```python
from build123d import *

# Parameters (mm, degrees)
SKETCH1_W           = 82
SKETCH1_H           = 82
BOSS_EXTRUDE3_DEPTH = 4
SKETCH6_W           = 10
SKETCH6_H           = 4
BOSS_EXTRUDE4_DEPTH = 12
CIRPATTERN1_COUNT   = 3
CIRPATTERN1_ANGLE   = 180
SKETCH8_W           = 4
SKETCH8_H           = 10
BOSS_EXTRUDE5_DEPTH = 85
SKETCH12_W          = 15.333160426
SKETCH12_H          = 4
BOSS_EXTRUDE6_DEPTH = 33
SKETCH9_W           = 7
SKETCH9_H           = 7
BOSS_EXTRUDE7_DEPTH = 4
SKETCH13_W          = 7
SKETCH13_H          = 7
BOSS_EXTRUDE8_DEPTH = 4


with BuildPart() as part:
    # Sketch1 → Boss-Extrude3 (new body)
    with BuildSketch(Plane.XY):
        Rectangle(SKETCH1_W, SKETCH1_H)
    extrude(amount=BOSS_EXTRUDE3_DEPTH)

    # Sketch6 → Boss-Extrude4 (add)
    with BuildSketch(Plane(origin=(0, 41, 0), x_dir=(1, 0, 0), z_dir=(0, 1, 0))):
        with Locations((0, -2)):
            Rectangle(SKETCH6_W, SKETCH6_H)
    boss_extrude4 = extrude(amount=BOSS_EXTRUDE4_DEPTH)

    # CirPattern1: Boss-Extrude4 ×3 about axis
    cirpattern1_axis = Axis((0, 0, 0), (0, 0, -1))
    for i in range(1, CIRPATTERN1_COUNT):
        add(boss_extrude4.rotate(cirpattern1_axis, i * CIRPATTERN1_ANGLE / (CIRPATTERN1_COUNT - 1)))

    # Sketch8 → Boss-Extrude5 (add)
    with BuildSketch(Plane.ZY.offset(41)):
        with Locations((2, 0)):
            Rectangle(SKETCH8_W, SKETCH8_H)
    extrude(amount=BOSS_EXTRUDE5_DEPTH)

    # Sketch12 → Boss-Extrude6 (add)
    with BuildSketch(Plane(origin=(0, 5, 0), x_dir=(1, 0, 0), z_dir=(0, 1, 0))):
        with Locations((-96, -2)):
            Rectangle(SKETCH12_W, SKETCH12_H)
    boss_extrude6 = extrude(amount=BOSS_EXTRUDE6_DEPTH)

    # Sketch9 → Boss-Extrude7 (add)
    with BuildSketch(Plane.XY.offset(4)):
        with Locations((-96, 0)):
            Rectangle(SKETCH9_W, SKETCH9_H)
    extrude(amount=BOSS_EXTRUDE7_DEPTH)

    # Sketch13 → Boss-Extrude8 (add)
    with BuildSketch(Plane.XY.offset(4)):
        with Locations((-96, 23.5)):
            Rectangle(SKETCH13_W, SKETCH13_H)
    boss_extrude8 = extrude(amount=BOSS_EXTRUDE8_DEPTH)

    # Mirror2: Boss-Extrude6, Boss-Extrude8 across plane
    add(boss_extrude6.mirror(Plane(origin=(0, 0, 0), x_dir=(0, 0, 1), z_dir=(0, -1, 0))))
    add(boss_extrude8.mirror(Plane(origin=(0, 0, 0), x_dir=(0, 0, 1), z_dir=(0, -1, 0))))


solid = part.part
```
Model file for the job. Use its own axes, mm. A direction names the side the tool comes from. Coordinates: 2 decimals unless noted, no trailing zeros. Order: outer loops, then holes, each group sorted by start corner. A loop starts at its lowest first (then second) coordinate and runs counter-clockwise, first axis right, second up. Notation, with made-up numbers: (25.5, -25.75) - (84.5, -25.75) arc R8 ccw to (84.5, -11.75) - close; hole circle Ø10 at (-23, 35). An arc over 180 degrees is marked (long way). Return JSON: item names as keys, results as strings. Group by question number.
1) Probe line 1 (Y direction, x = -94, z = 4.5); line 2 (X direction, y = -15, z = 3); line 3 (Z direction, x = -32.5, y = 26.5). List the from-to ranges inside material, lowest first. Write a range as from..to.
2) Flat gauge pins, fed straight in: P1, Ø3, axis at x = 9, z = 3.5, coming from the -Y side; P2, Ø4.5, axis at y = -15.5, z = 2, coming from the +X side; P3, Ø2, axis at y = -28.5, z = 1.5, coming from the -X side; P4, Ø3, axis at y = 38.5, z = 6, coming from the -X side. Where does each tip first touch, or does it go through?
3) Saw through at B-B, the plane z = 5.5. Write the cut outline in (x, y).
4) Saw through at D-D, the plane x = -94.5. Write the cut outline in (y, z), plus the area to 3 significant figures.
5) Mould opens along Y. For faces 1 (the flat face through (23, 41, 2)), 2 (the flat face through (-96, -20, 6)), 3 (the flat face through (-126, 0, 2)) say: released by +Y, released by -Y, zero draft, split by the parting line, or undercut.
6) Saw through at C-C, the plane y = -1.5. Write the cut outline in (x, z), plus the area to 3 significant figures.
7) Tool access for faces 4 (the flat face through (-99.5, -23, 6)), 5 (the flat face through (-96, 3.5, 6)), 6 (the flat face through (-5, 47, 2)): list every direction of +Z, -Z, +X, -X, +Y, -Y with a clear straight run to the whole face (end or side of a thin tool).
8) Saw through at A-A, the plane y = 11.5. Write the cut outline in (x, z).
Values found:
{
 "1": {"line 1": "y = -27..-20, -3.5..3.5, 20..27", "line 2": "x = -103.67..-88.33, -41..41", "line 3": "z = 0..4"},
 "2": {"P1": "stops at y = -41", "P2": "stops at x = 41", "P3": "stops at x = -103.67", "P4": "passes through"},
 "3": {"outline": "(-99.5, -27) - (-92.5, -27) - (-92.5, -20) - (-99.5, -20) - close; (-99.5, -3.5) - (-92.5, -3.5) - (-92.5, 3.5) - (-99.5, 3.5) - close; (-99.5, 20) - (-92.5, 20) - (-92.5, 27) - (-99.5, 27) - close"},
 "4": {"outline": "(-38, 0) - (38, 0) - (38, 4) - (27, 4) - (27, 8) - (20, 8) - (20, 4) - (3.5, 4) - (3.5, 8) - (-3.5, 8) - (-3.5, 4) - (-20, 4) - (-20, 8) - (-27, 8) - (-27, 4) - (-38, 4) - close", "area": "388 mm²"},
 "5": {"face 1": "released by +Y", "face 2": "undercut", "face 3": "zero draft"},
 "6": {"outline": "(-126, 0) - (53, 0) - (53, 4) - (-92.5, 4) - (-92.5, 8) - (-99.5, 8) - (-99.5, 4) - (-126, 4) - close", "area": "744 mm²"},
 "7": {"face 4": "+Z, -X, +Y, -Y", "face 5": "+Z, +X, -X", "face 6": "+Z, -Z, -X, +Y"},
 "8": {"outline": "(-103.67, 0) - (-88.33, 0) - (-88.33, 4) - (-103.67, 4) - close; (-41, 0) - (41, 0) - (41, 4) - (-41, 4) - close"}
}
